The model under review builds one solid part; all positions refer to its coordinate system, in mm. A direction names the side the tool comes from. Give positions to 0.01 mm unless a question says otherwise; leave off trailing zeros. Write each loop counter-clockwise with the first axis right and the second up, starting at its lowest first coordinate (ties: lowest second). Pieces come first, ordered by that corner, then holes. Notation, with made-up numbers: (11.25, 79.5) - (21.25, 79.5) arc R7 ccw to (21.25, 84.5) - close; hole circle Ø1 at (-18, -29). An arc over 180 degrees is marked (long way). One line per question, with ' | ' between items. Start each with the question number.
```python
from build123d import *

# Parameters (mm, degrees)
SKETCH1_W           = 59.45
SKETCH1_H           = 33.05
BOSS_EXTRUDE1_DEPTH = 10
CUT_EXTRUDE1_DEPTH  = 1.72
SKETCH3_W           = 54.45
SKETCH3_H           = 4.5
CUT_EXTRUDE2_DEPTH  = 9.2


with BuildPart() as part:
    # Sketch1 → Boss-Extrude1 (new body)
    with BuildSketch(Plane(origin=(0, 0, 0), x_dir=(1, 0, 0), z_dir=(0, 1, 0))):
        Rectangle(SKETCH1_W, SKETCH1_H)
    extrude(amount=BOSS_EXTRUDE1_DEPTH)

    # Sketch2 → Cut-Extrude1 (cut)
    with BuildSketch(Plane(origin=(0, 10, 0), x_dir=(1, 0, 0), z_dir=(0, 1, 0))):
        Polygon((-27.225, -4.275), (-29.72540031, -4.275), (-29.725, 4.584999991), (-27.225, 4.584999991), (-27.225, 14.025), (27.225, 14.025), (27.225, -14.025), (-27.225, -14.025), align=None)
    extrude(amount=-CUT_EXTRUDE1_DEPTH, mode=Mode.SUBTRACT)

    # Sketch3 → Cut-Extrude2 (cut)
    with BuildSketch(Plane(origin=(0, 8.28, 0), x_dir=(1, 0, 0), z_dir=(0, 1, 0))):
        with Locations((0, 11.775)):
            Rectangle(SKETCH3_W, SKETCH3_H)
        with Locations((0, -11.775)):
            Rectangle(SKETCH3_W, SKETCH3_H)
    extrude(amount=-CUT_EXTRUDE2_DEPTH, mode=Mode.SUBTRACT)


solid = part.part
```
Item 1: Take a section at A-A (y = 1.75). Give the boundary of the cut face in (x, z) (3 decimals), plus the area to 3 significant figures.
Item 2: Take a section at D-D (z = -6). Give the boundary of the cut face in (x, y) (3 decimals).
Item 3: Take a section at B-B (x = -15). Give the boundary of the cut face in (y, z) (3 decimals).
Item 4: The part is to be moulded in two halves that separate along Z. For faces 4 (the flat face through (-29.725, 5, 0)), 5 (the flat face through (0, 5, -16.525)), 6 (the flat face through (27.225, 9.5, 3.3)), 7 (the flat face through (0, 5, 16.525)), say which applies: +Z half, -Z half, draft (parallel to the pull), parting line (faces both ways), or undercut.
Item 5: Machinability: for faces 1 (the flat face through (-28, 9, -4.585)), 2 (the flat face through (-27.225, 6, 11)), 3 (the flat face through (0, 5, -14.025)), which of the approach directions +Z, -Z, +X, -X, +Y, -Y give a long, thin tool a straight path to every point of the face, cutting with its end or side? Answer none if there is none.
Item 6: Clearance check with a flat-ended pin moving along its axis: P1, Ø5.5, axis at x = 2, z = -2, coming from the +Y side. State where the tip first meets the part, or that it passes through.
Item 7: For probe 1 along Z at (x, y) = (-20.5, 7.5) (3 decimals); probe 2 along X at (y, z) = (1.75, -12.5) (3 decimals); probe 3 along Z at (x, y) = (-1, 8.75) (3 decimals), list the stretches that pass through material, from the lowest coordinate up.
Item 8: Take a section at C-C (z = -12). Give the boundary of the cut face in (x, y) (3 decimals).
Check sheet entries:
1) outline: (-29.725, -16.525) - (29.725, -16.525) - (29.725, 16.525) - (-29.725, 16.525) - close; hole (-27.225, -14.025) - (27.225, -14.025) - (27.225, -9.525) - (-27.225, -9.525) - close; hole (-27.225, 9.525) - (27.225, 9.525) - (27.225, 14.025) - (-27.225, 14.025) - close | area: 1,470 mm^2
2) outline: (-29.725, 0) - (29.725, 0) - (29.725, 10) - (27.225, 10) - (27.225, 8.28) - (-27.225, 8.28) - (-27.225, 10) - (-29.725, 10) - close
3) outline: (0, -16.525) - (10, -16.525) - (10, -14.025) - (0, -14.025) - close; (0, -9.525) - (8.28, -9.525) - (8.28, 9.525) - (0, 9.525) - close; (0, 14.025) - (10, 14.025) - (10, 16.525) - (0, 16.525) - close
4) face 4: draft | face 5: -Z half | face 6: undercut | face 7: +Z half
5) face 1: -X, +Y | face 2: +Y | face 3: +Y, -Y
6) P1: stops at y = 8.28
7) probe 1: z = -16.525 to -14.025, -9.525 to 9.525, 14.025 to 16.525 | probe 2: x = -29.725 to -27.225, 27.225 to 29.725 | probe 3: z = -16.525 to -14.025, 14.025 to 16.525
8) outline: (-29.725, 0) - (-27.225, 0) - (-27.225, 10) - (-29.725, 10) - close; (27.225, 0) - (29.725, 0) - (29.725, 10) - (27.225, 10) - close
